Solid Edge part; units mm, degrees
sketch "Sketch1" plane through (0, 0, 0) normal (0, -1, 0) x (1, 0, 0)
  line L0 (-6.5, 15) -> (6.5, 15)
  line L1 (6.5, 15) -> (6.5, -15)
  line L2 (6.5, -15) -> (-6.5, -15)
  line L3 (-6.5, -15) -> (-6.5, 15)
  dimension "D1" = 6.5
  dimension "D2" = 6.5
extrude "Ajout_matière_1" add sketch "Sketch1" along normal mid plane 12
sketch "Sketch2" plane through (0, 6, 0) normal (0, 1, 0) x (-1, 0, 0)
  line L0 (-4, 12.5) -> (-4, -12.5)
  line L1 (-4, -12.5) -> (4, -8.8636)
  line L2 (4, -8.8636) -> (4, 8.8636)
  line L3 (4, 8.8636) -> (-4, 12.5)
  dimension "D1" = 4
  dimension "D2" = 4
extrude "Cutout1" cut sketch "Sketch2" against normal up to next
sketch "Sketch3" plane through (0, 0, 15) normal (0, 0, 1) x (1, 0, 0)
  line L0 (-6.5, 0) -> (6.5, 0)
  line L1 (6.5, 0) -> (6.5, -6)
  line L2 (6.5, -6) -> (-6.5, -6)
  line L3 (-6.5, -6) -> (-6.5, 0)
extrude "Protrusion1" add sketch "Sketch3" along normal blind 12 and the other way blind 1
hole "Perçage_2" at (0, 0, 21) direction (0, -1, 0) diameter 5.3 end up to next countersink diameter 11.47 countersink angle 90
mirror "Mirror1" about plane through (0, 0, 0) normal (0, 0, 1) of "Protrusion1", "Perçage_2"
hole "Perçage_4" at (-6.5, 0, 0) direction (1, 0, 0) diameter 5 end up to next
chamfer "Chanfrein_1" distance 0.5 angle 45 18 edges at (0, 6, 15) (6.5, 6, 0) (-6.5, 6, 0) (0, 6, -15) (-6.5, 3, 15) (-6.5, 3, -15) (-6.5, 0, -21) (6.5, 3, 15) (6.5, 3, -15) (6.5, 0, -21) (0, 0, -27) (6.5, 0, 21) (0, 0, 27) (-6.5, 0, 21) (6.5, -3, 27) (-6.5, -3, 27) (6.5, -3, -27) (-6.5, -3, -27)
properties material "Aluminium AU4G, 2024_T4"
Geometry: final body of the model. Coordinates: model frame, mm. A direction names the side the tool comes from. Round coordinates to 2 decimals unless told otherwise and drop trailing zeros. Write each loop counter-clockwise with the first axis right and the second up, starting at its lowest first coordinate (ties: lowest second). Pieces come first, ordered by that corner, then holes.
Item 1: Section query C-C (z = 21). Return loops of the section in (x, y) (3 decimals).
Item 2: Material intervals for L1, parallel to Y at x = -4.9, z = 0; L2, parallel to X at y = -3.9, z = -21; L3, parallel to X at y = 2.25, z = 5.5, sorted ascending.
Item 3: Section query B-B (y = 4.5). Return loops of the section in (x, z), plus the area to 3 significant figures.
Item 4: Section query A-A (z = 0). Return loops of the section in (x, y), plus the area to 4 significant figures.
Item 5: Section query D-D (y = -5). Return loops of the section in (x, z).
Item 6: Set-up query: faces 4 (the face through (0, 3, 15)), 5 (the face through (0, -3, 27)), 6 (the face through (0, 3, -15)), 7 (the face through (-0.056, 0.084, 10.656)), 8 (the face through (-5.27, -2.44, -0.54)). Return all of +Z, -Z, +X, -X, +Y, -Y with unobstructed straight access to the full face (end or side cutting, diameter ignored); none if empty.
Item 7: Pin query (flat end, axial travel): P1, Ø3, axis at x = 3, z = 9, coming from the -Y side; P2, Ø4.5, axis at y = 0, z = 0, coming from the -X side; P3, Ø4.5, axis at x = 2.5, y = 2, coming from the -Z side; P4, Ø1.6, axis at x = -2, y = 4, coming from the +Z side. Return the tip coordinate at first contact, or that it passes through.
Item 8: Mould query, pull axis X, two halves, no side actions, for faces 1 (the face through (-6.5, -3, 0)), 2 (the face through (0.854, -2.892, 23.712)), 3 (the face through (5, 6, 0)). Classes: +X half, -X half, draft (parallel to the pull), parting line (faces both ways), or undercut.
Completed:
1. outline: (-6.5, -6) - (-2.65, -6) - (-2.65, -3.085) - (-5.735, 0) - (-6, 0) - (-6.5, -0.5) - close; (2.65, -6) - (6.5, -6) - (6.5, -0.5) - (6, 0) - (5.735, 0) - (2.65, -3.085) - close
2. L1: y = -6 to -2.5, 2.5 to 6
2. L2: x = -6.5 to -2.65, 2.65 to 6.5
2. L3: x = -6.5 to -4, 4 to 6.5
3. outline: (-6.5, -14.5) - (-6, -15) - (6, -15) - (6.5, -14.5) - (6.5, 14.5) - (6, 15) - (-6, 15) - (-6.5, 14.5) - close; hole (-4, -8.86) - (4, -12.5) - (4, 12.5) - (-4, 8.86) - close
3. area: 219 mm2
4. outline: (-6.5, -6) - (-4, -6) - (-4, -2.5) - (-6.5, -2.5) - close; (-6.5, 2.5) - (-4, 2.5) - (-4, 6) - (-6, 6) - (-6.5, 5.5) - close; (4, -6) - (6.5, -6) - (6.5, 5.5) - (6, 6) - (4, 6) - close
4. area: 47.25 mm2
5. outline: (-6.5, -26.5) - (-6, -27) - (6, -27) - (6.5, -26.5) - (6.5, 26.5) - (6, 27) - (-6, 27) - (-6.5, 26.5) - close; hole (-4, -8.86) - (4, -12.5) - (4, 12.5) - (-4, 8.86) - close; hole circle Ø5.3 at (0, -21); hole circle Ø5.3 at (0, 21)
6. face 4: +Z, +X, -X, +Y
6. face 5: +Z, +X, -X, +Y, -Y
6. face 6: -Z, +X, -X, +Y
6. face 7: +Y, -Y
6. face 8: -X
7. P1: stops at y = -6
7. P2: stops at x = 4
7. P3: stops at z = -26.75
7. P4: stops at z = 15
8. face 1: -X half
8. face 2: undercut
8. face 3: draft
